```python
from build123d import *

# Parameters (mm, degrees)
CUT_EXTRUDE1_DEPTH = 1.5


with BuildPart() as part:
    # Sketch1 → Revolve1 (revolve)
    with BuildSketch(Plane.XY):
        with BuildLine():
            Line((0, 0), (20, 0))
            Line((20, 0), (20, -1.5))
            Line((20, -1.5), (-2, -1.5))
            Line((-2, -1.5), (-2, 0))
            ThreePointArc((-2, 0), (-1.356037029, 0.752244435), (-0.5, 1.25))
            ThreePointArc((-0.5, 1.25), (-0.192181086, 1.122273642), (0, 0.85))
            Line((0, 0.85), (0, 0))
        make_face()
    revolve(axis=Axis((20, -1.5, 0), (-1, 0, 0)))

    # Sketch2 → Cut-Extrude1 (cut)
    with BuildSketch(Plane.ZY.offset(2)):
        Polygon((0, -0.229829408), (-1.1, -0.864914704), (-1.1, -2.135085296), (0, -2.770170592), (1.1, -2.135085296), (1.1, -0.864914704), align=None)
    extrude(amount=-CUT_EXTRUDE1_DEPTH, mode=Mode.SUBTRACT)


solid = part.part
```
The listing builds one solid part. Answer for the finished solid, in the listing's coordinates (mm). A direction names the side the tool comes from. Round coordinates to 2 decimals unless told otherwise and drop trailing zeros. Loops run counter-clockwise (first coordinate to the right, second up) from the corner with the lowest first, then second, coordinate; pieces in that order, holes last.
Q1. Find the intervals of material crossed by line 1 (X direction, y = -1.4, z = 0.15); line 2 (Z direction, x = 16, y = -1.55); line 3 (Y direction, x = -0.75, z = -2.4), in increasing order.
Q2. For a pull along Z with two mould halves and no side action, classify faces 3 (the face through (0, -2, 2)), 4 (the face through (-1.3, -1.5, -1.1)), 5 (the face through (-1.3, -1.5, 1.1)), 6 (the face through (10.1, -2.7, 0.9)) as released by +Z, released by -Z, zero draft, split by the parting line, or undercut.
Q3. Which of the six approach directions +Z, -Z, +X, -X, +Y, -Y give full straight-line access (tool end or side, diameter ignored) to faces 1 (the face through (-1.26, -2.448, -0.558)), 2 (the face through (20, -2, 0))?
Q4. Given pin 1 Ø0.6 at (x, y) = (-1, -1.5) entering from +Z; pin 2 Ø1 at (x, y) = (17.5, 0) entering from +Z; pin 3 Ø1.1 at (y, z) = (-1.5, -0.5) entering from -X, each flat-ended and moving along its own axis, determine where each tip first touches the part or whether it passes through.
Q5. Section A-A, the plane x = 18.25 is taken. Determine the outline of the cut face in (y, z).
Completed:
1. line 1: x = -0.5 to 20
1. line 2: z = -1.5 to 1.5
1. line 3: y = -2.61 to -0.39
2. face 3: zero draft
2. face 4: undercut
2. face 5: undercut
2. face 6: split by the parting line
3. face 1: -X
3. face 2: +Z, -Z, +X, +Y, -Y
4. pin 1: stops at z = 2.67
4. pin 2: stops at z = 1.12
4. pin 3: stops at x = -0.5
5. outline: circle Ø3 at (-1.5, 0)
